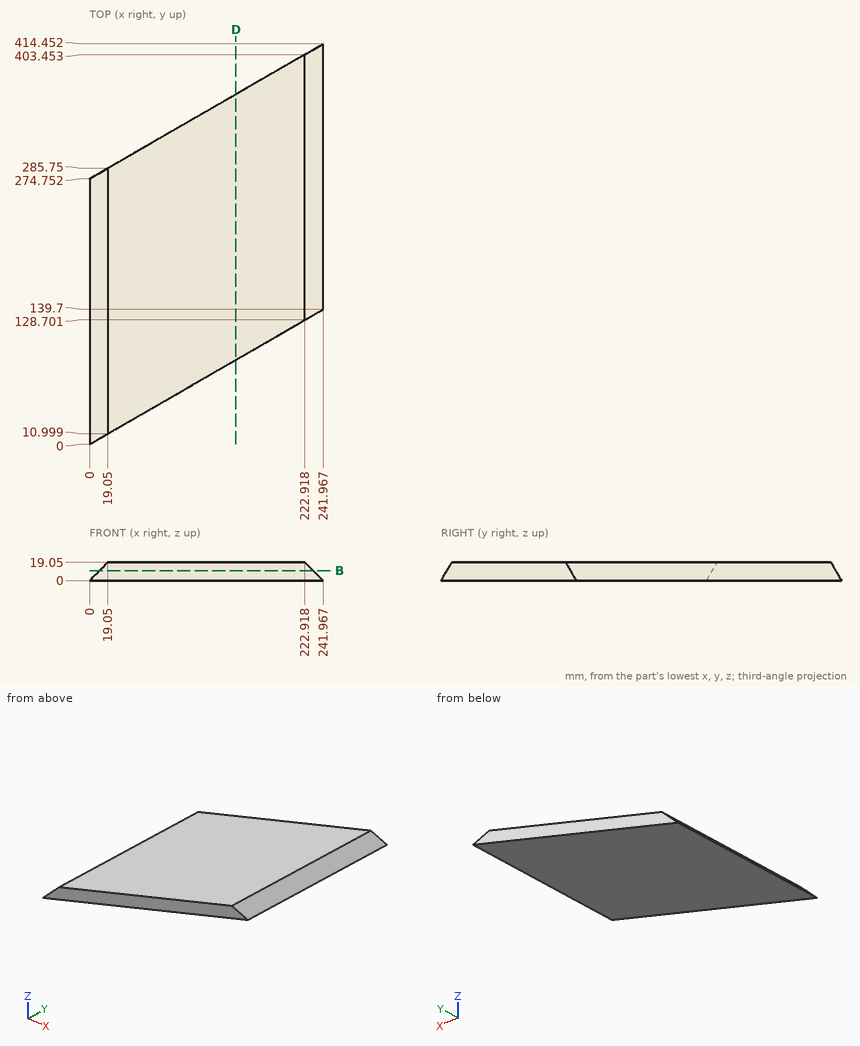
Geometry check sheet. Reference: drawing and pictorial views, mm from the part's lowest x, y, z. Give positions to 0.01 mm unless a question says otherwise; leave off trailing zeros. Write each loop counter-clockwise with the first axis right and the second up, starting at its lowest first coordinate (ties: lowest second). Pieces come first, ordered by that corner, then holes. Notation, with made-up numbers: (68.25, 44.25) - (91.25, 44.25) arc R16 cw to (91.25, 52.25) - close; hole circle Ø5 at (29, 66.5). An arc over 180 degrees is marked (long way). Use a Markdown table: item, result.
Q1. Thickness scan on L1, parallel to Y at x = 97.5, z = 14 (1 decimal); L2, parallel to X at y = 139.5, z = 3.5 (1 decimal); L3, parallel to Y at x = 92.5, z = 16.5 (1 decimal). Record the ranges inside material, lowest first. Write a range as [from, to].
Computed:
| item | result |
|---|---|
| L1 | y = [56.3, 331] |
| L2 | x = [3.5, 238.5] |
| L3 | y = [53.4, 328.2] |
Q2. Section check D-D, the plane x = 151.5. Enter the section's corners in (y, z), then the cut area to 3 significant figures.
Computed:
| item | result |
|---|---|
| outline | (87.47, 0) - (362.22, 0) - (362.22, 19.05) - (87.47, 19.05) - close |
| area | 5,230 mm² |
Q3. Go/stop test with flat-tipped pins: P1, Ø3, axis at y = 296.5, z = 14.5, coming from the -X side; P2, Ø4, axis at x = 67, z = 11.5, coming from the +Y side; P3, Ø6, axis at y = 171.5, z = 16, coming from the +X side. Record where each tip stops, or that it passes through.
Computed:
| item | result |
|---|---|
| P1 | stops at x = 35.07 |
| P2 | stops at y = 314.59 |
| P3 | stops at x = 228.97 |
Q4. Section check B-B, the plane z = 10.5. Enter the section's corners in (x, y), then the cut area to 3 significant figures.
Computed:
| item | result |
|---|---|
| outline | (10.5, 6.06) - (231.47, 133.64) - (231.47, 408.39) - (10.5, 280.81) - close |
| area | 60,700 mm² |
